Geometry: see drawing. Coordinates: mm, zero at the bounding-box minimum. Give positions to 0.01 mm unless a question says otherwise; leave off trailing zeros. Loops run counter-clockwise (first coordinate to the right, second up) from the corner with the lowest first, then second, coordinate; pieces in that order, holes last. Notation, with made-up numbers: (27, 86) -> (42, 86) arc R27 cw to (42, 108) -> close; hole circle Ø9 at (84, 59.25). An arc over 180 degrees is marked (long way). Return JSON: item names as keys, results as strings. Group by question number.
(1) Pin query (flat end, axial travel): pin 1 (1.5 mm diameter, centred on x = 0.5, z = 4, fed in from +Y). Return the tip coordinate at first contact, or that it passes through.
(2) Cut plane C-C on z = 3.85. Return loops of the section in (x, y).
(3) Draft query along X for the marked faces 1, 2 and 3. Return one class per face: released by +X, released by -X, zero draft, split by the parting line, or undercut.
(4) Cut plane A-A on x = 2.3. Return loops of the section in (y, z).
(5) Ray query, line 1 (Y direction, x = 2.3, z = 2.2); line 2 (Y direction, x = 3.55, z = 3.15). Return the intervals inside material, ascending. Write a range as from..to.
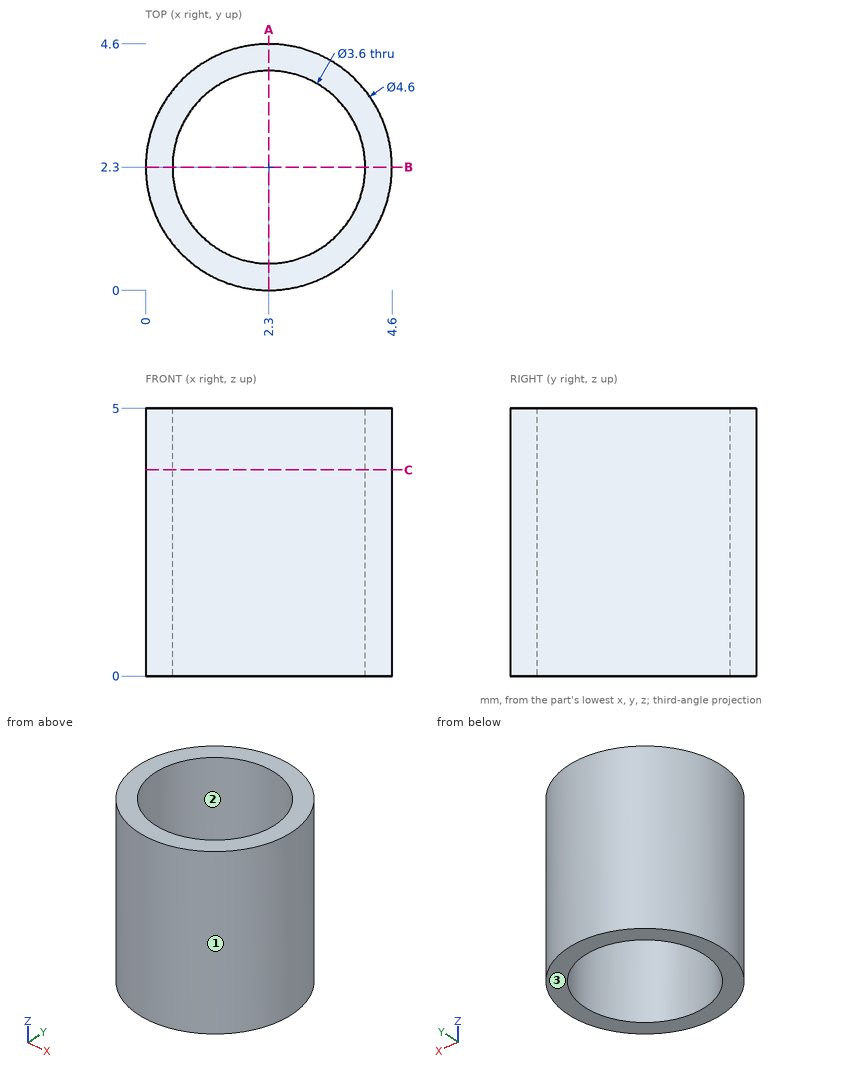
Answers:
{
 "1": {"pin 1": "y = 4.35"},
 "2": {"outline": "circle Ø4.6 at (2.3, 2.3); hole circle Ø3.6 at (2.3, 2.3)"},
 "3": {"face 1": "split by the parting line", "face 2": "undercut", "face 3": "zero draft"},
 "4": {"outline": "(0, 0) -> (0.5, 0) -> (0.5, 5) -> (0, 5) -> close; (4.1, 0) -> (4.6, 0) -> (4.6, 5) -> (4.1, 5) -> close"},
 "5": {"line 1": "0..0.5, 4.1..4.6", "line 2": "0.37..1, 3.6..4.23"}
}
